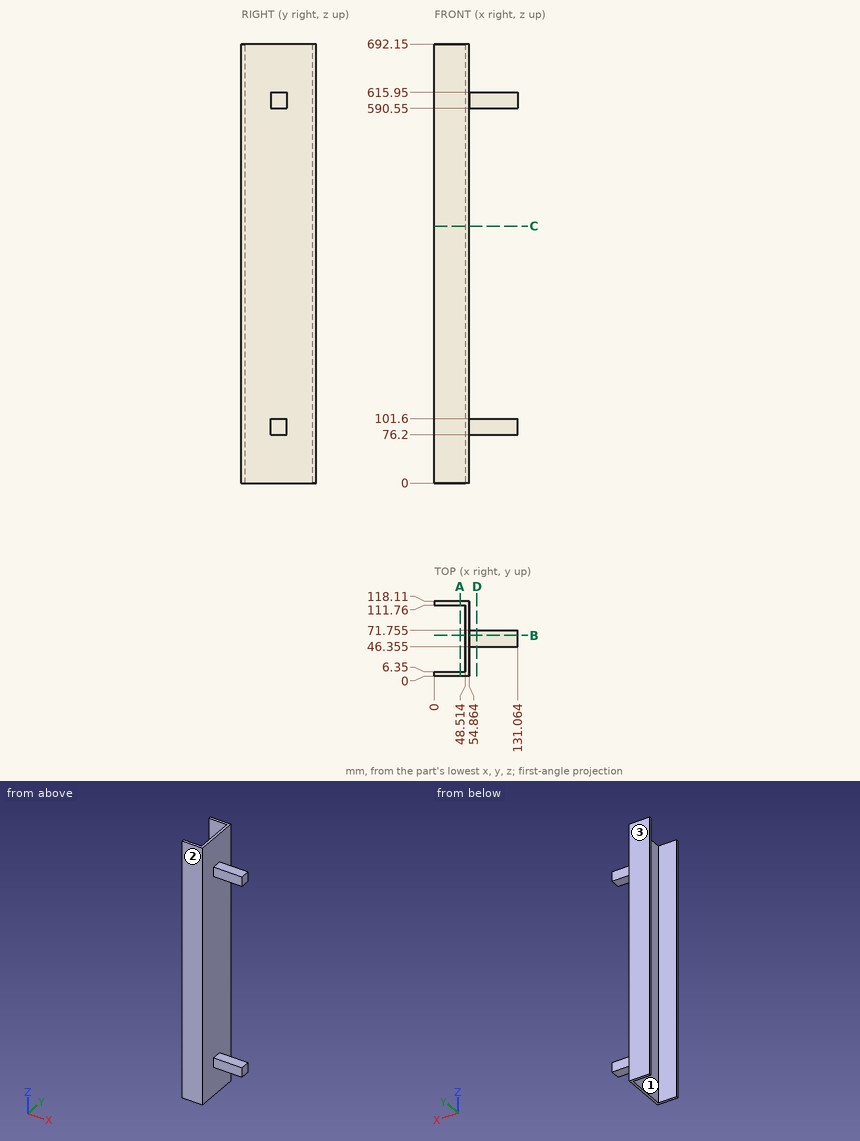
Study the drawing (mm; zero at the part's minimum x, y, z) and answer. Round coordinates to 2 decimals unless told otherwise and drop trailing zeros. Order: outer loops, then holes, each group sorted by start corner. A loop starts at its lowest first (then second) coordinate and runs counter-clockwise, first axis right, second up. Notation, with made-up numbers: M 54.5,73.25 L 109.5,73.25 A21 cw 109.5,110.25 Z; hole C -7.75,54 d9. An arc over 180 degrees is marked long. One line per item, written item: value.
Q1. Find section D-D on x = 67. Write down the section's boundary in (y, z) (3 decimals), then the cut area to 3 significant figures.
Derived:
outline: M 46.355,76.2 L 71.755,76.2 L 71.755,101.6 L 46.355,101.6 Z; M 46.355,590.55 L 71.755,590.55 L 71.755,615.95 L 46.355,615.95 Z
area: 1,290 mm²
Q2. Straight lines are drawn through the part: line 1 (Y direction, x = 39, z = 95); line 2 (Z direction, x = 73.5, y = 55.5); line 3 (X direction, y = 57, z = 590). For each, find the intervals that lie inside material, in ascending order.
Derived:
line 1: 0 to 6.35, 111.76 to 118.11
line 2: 76.2 to 101.6, 590.55 to 615.95
line 3: 48.51 to 54.86
Q3. Flat-ended cylindrical pins translate along their axes: pin 1 (3 mm diameter, centred on x = 77.5, y = 64, fed in from -Z); pin 2 (1.5 mm diameter, centred on y = 85.5, z = 74, fed in from -X); pin 3 (20.5 mm diameter, centred on x = 76.5, z = 601.5, fed in from +Y) (3 decimals); pin 4 (8 mm diameter, centred on x = 60.5, y = 85, fed in from -Z). Find the tip coordinate at first contact, or state that the pin passes through.
Derived:
pin 1: z = 76.2
pin 2: x = 48.51
pin 3: y = 71.755
pin 4: through
Q4. Determine the mould class of the marked faces 1, 2 and 3 for opening direction Y: released by +Y, released by -Y, zero draft, split by the parting line, or undercut.
Derived:
face 1: undercut
face 2: released by -Y
face 3: released by +Y
Q5. Find section A-A on x = 40.5. Write down the section's boundary in (y, z), then the cut area to 3 significant figures.
Derived:
outline: M 0,0 L 6.35,0 L 6.35,692.15 L 0,692.15 Z; M 111.76,0 L 118.11,0 L 118.11,692.15 L 111.76,692.15 Z
area: 8,790 mm²
Q6. Find section C-C on z = 405. Write down the section's boundary in (x, y).
Derived:
outline: M 0,0 L 54.86,0 L 54.86,118.11 L 0,118.11 L 0,111.76 L 48.51,111.76 L 48.51,6.35 L 0,6.35 Z
Q7. Find section B-B on y = 64. Write down the section's boundary in (x, z), then the cut area to 3 significant figures.
Derived:
outline: M 48.51,0 L 54.86,0 L 54.86,76.2 L 131.06,76.2 L 131.06,101.6 L 54.86,101.6 L 54.86,590.55 L 131.06,590.55 L 131.06,615.95 L 54.86,615.95 L 54.86,692.15 L 48.51,692.15 Z
area: 8,270 mm²
